from build123d import *

# Parameters (mm, degrees)
CYLINDER002_R     = 18
CYLINDER002_DEPTH = 76
CYLINDER003_R     = 18
CYLINDER003_DEPTH = 76
CYLINDER004_R     = 18
CYLINDER004_DEPTH = 76
CYLINDER005_R     = 18
CYLINDER005_DEPTH = 76
CYLINDER_R        = 18
CYLINDER_DEPTH    = 76
CYLINDER001_R     = 18
CYLINDER001_DEPTH = 76
BOX_W             = 230
BOX_H             = 110
BOX_DEPTH         = 76


with BuildPart() as cilindro002:
    # Cylinder002 → Cylinder002 (new body)
    with BuildSketch(Plane(origin=(43, 31, 0), x_dir=(1, 0, 0), z_dir=(0, 0, 1))):
        Circle(CYLINDER002_R)
    extrude(amount=CYLINDER002_DEPTH)


with BuildPart() as fusion001:
    # Cylinder003 → Cylinder003 (new body)
    with BuildSketch(Plane(origin=(43, 79, 0), x_dir=(1, 0, 0), z_dir=(0, 0, 1))):
        Circle(CYLINDER003_R)
    extrude(amount=CYLINDER003_DEPTH)

    # Fusion001: union Cilindro002
    add(cilindro002.part)


with BuildPart() as fusion001_1:
    # Fusion001 placement: moved
    add(fusion001.part.moved(Location((72, 0, 0))))


with BuildPart() as cilindro004:
    # Cylinder004 → Cylinder004 (new body)
    with BuildSketch(Plane(origin=(43, 31, 0), x_dir=(1, 0, 0), z_dir=(0, 0, 1))):
        Circle(CYLINDER004_R)
    extrude(amount=CYLINDER004_DEPTH)


with BuildPart() as fusion002:
    # Cylinder005 → Cylinder005 (new body)
    with BuildSketch(Plane(origin=(43, 79, 0), x_dir=(1, 0, 0), z_dir=(0, 0, 1))):
        Circle(CYLINDER005_R)
    extrude(amount=CYLINDER005_DEPTH)

    # Fusion002: union Cilindro004
    add(cilindro004.part)


with BuildPart() as fusion002_1:
    # Fusion002 placement: moved
    add(fusion002.part.moved(Location((144, 0, 0))))


with BuildPart() as cilindro:
    # Cylinder → Cylinder (new body)
    with BuildSketch(Plane(origin=(43, 31, 0), x_dir=(1, 0, 0), z_dir=(0, 0, 1))):
        Circle(CYLINDER_R)
    extrude(amount=CYLINDER_DEPTH)


with BuildPart() as fusion:
    # Cylinder001 → Cylinder001 (new body)
    with BuildSketch(Plane(origin=(43, 79, 0), x_dir=(1, 0, 0), z_dir=(0, 0, 1))):
        Circle(CYLINDER001_R)
    extrude(amount=CYLINDER001_DEPTH)

    # Fusion: union Cilindro
    add(cilindro.part)


with BuildPart() as cut002:
    # Box → Box (new body)
    with BuildSketch(Plane.XY):
        with Locations((115, 55)):
            Rectangle(BOX_W, BOX_H)
    extrude(amount=BOX_DEPTH)

    # Cut: cut Fusion
    add(fusion.part, mode=Mode.SUBTRACT)

    # Cut001: cut Fusion002
    add(fusion002_1.part, mode=Mode.SUBTRACT)

    # Cut002: cut Fusion001
    add(fusion001_1.part, mode=Mode.SUBTRACT)


solid = cut002.part
Can you work these out from the model? Positions are in its coordinate system, mm. Give positions to 0.01 mm unless a question says otherwise; leave off trailing zeros. Loops run counter-clockwise (first coordinate to the right, second up) from the corner with the lowest first, then second, coordinate; pieces in that order, holes last. Notation, with made-up numbers: (-21.75, 2.5) - (37.25, 2.5) arc R18 ccw to (37.25, 37.5) - close; hole circle Ø5 at (-39.5, 3.25). An arc over 180 degrees is marked (long way). Answer as a JSON object with one key per item and string values.
Q1. Imagine slicing it at C-C on z = 6. Write out the boundary of the cut face in (x, y), plus the area to 3 significant figures.
Geometry says:
{"outline": "(0, 0) - (230, 0) - (230, 110) - (0, 110) - close; hole circle Ø36 at (43, 31); hole circle Ø36 at (43, 79); hole circle Ø36 at (115, 31); hole circle Ø36 at (115, 79); hole circle Ø36 at (187, 31); hole circle Ø36 at (187, 79)", "area": "19,200 mm²"}
Q2. Will this pin go through, and if not, where does the flat tip stop? P1, Ø1, axis at y = 92.5, z = 22, coming from the -X side.
Geometry says:
{"P1": "x = 0"}
Q3. Imagine slicing it at D-D on y = 39. Write out the boundary of the cut face in (x, z), plus the area to 3 significant figures.
Geometry says:
{"outline": "(0, 0) - (26.88, 0) - (26.88, 76) - (0, 76) - close; (59.12, 0) - (98.88, 0) - (98.88, 76) - (59.12, 76) - close; (131.12, 0) - (170.88, 0) - (170.88, 76) - (131.12, 76) - close; (203.12, 0) - (230, 0) - (230, 76) - (203.12, 76) - close", "area": "10,100 mm²"}
Q4. If I drill on L1, parallel to Y at x = 187, z = 26.5; L2, parallel to X at y = 67.5, z = 67; L3, parallel to X at y = 41, z = 56.5, over which ranges is the centre line in solid material (lowest first)?
Geometry says:
{"L1": "0 to 13, 49 to 61, 97 to 110", "L2": "0 to 29.15, 56.85 to 101.15, 128.85 to 173.15, 200.85 to 230", "L3": "0 to 28.03, 57.97 to 100.03, 129.97 to 172.03, 201.97 to 230"}
Q5. Imagine slicing it at B-B on y = 79. Write out the boundary of the cut face in (x, z).
Geometry says:
{"outline": "(0, 0) - (25, 0) - (25, 76) - (0, 76) - close; (61, 0) - (97, 0) - (97, 76) - (61, 76) - close; (133, 0) - (169, 0) - (169, 76) - (133, 76) - close; (205, 0) - (230, 0) - (230, 76) - (205, 76) - close"}
Q6. If we mould it in two halves opening along Y, with no side actions, what happens to faces 1 (the flat face through (113, 0, 37)), 2 (the flat face through (113, 56, 76)), 3 (the cylindrical face through (203.63, 24.11, 37.47))? For each: pulls with the +Y half, pulls with the -Y half, needs draft (parallel to the pull), parting line crosses it, or undercut.
Geometry says:
{"face 1": "pulls with the -Y half", "face 2": "needs draft", "face 3": "undercut"}
Q7. Imagine slicing it at A-A on x = 43. Write out the boundary of the cut face in (y, z), plus the area to 3 significant figures.
Geometry says:
{"outline": "(0, 0) - (13, 0) - (13, 76) - (0, 76) - close; (49, 0) - (61, 0) - (61, 76) - (49, 76) - close; (97, 0) - (110, 0) - (110, 76) - (97, 76) - close", "area": "2,890 mm²"}
